```python
from build123d import *

# Parameters (mm, degrees)
F1_DEPTH = 6.858
F2_R     = 2.54
F3_R     = 1.723698
F4_DEPTH = 13.6906


with BuildPart() as f1:
    # F0 (on Top) → F1 (new body)
    with BuildSketch(Plane.XY):
        Polygon((-21.122105, 0), (0, 0), (21.122105, 0), (21.122105, 49.931053), (13.769474, 49.931053), (13.769474, 6.35), (0, 6.35), (-13.769474, 6.35), (-13.769474, 49.931053), (-21.122105, 49.931053), align=None)
    extrude(amount=F1_DEPTH)

    # F2
    f2_edges = [f1.edges().sort_by_distance(p)[0] for p in [
        (13.769474, 28.140527, 0),
        (0, 6.35, 0),
        (-13.769474, 28.140527, 0),
        (0, 0, 6.858),
        (21.122105, 0, 3.429),
        (21.122105, 49.931053, 3.429),
        (21.122105, 24.965527, 6.858),
        (-21.122105, 0, 3.429),
        (-21.122105, 24.965527, 0),
        (-21.122105, 24.965527, 6.858),
        (0, 0, 0),
        (21.122105, 24.965527, 0),
        (-13.769474, 28.140527, 6.858),
        (0, 6.35, 6.858),
    ]]
    fillet(f2_edges, radius=F2_R)

    # F3 (on face) → F4 (join)
    with BuildSketch(Plane(origin=(0, 49.931053, 0), x_dir=(-1, 0, 0), z_dir=(0, 1, 0))):
        with Locations((17.637752, 3.690227)):
            Circle(F3_R)
    extrude(amount=-F4_DEPTH)


solid = f1.part
```
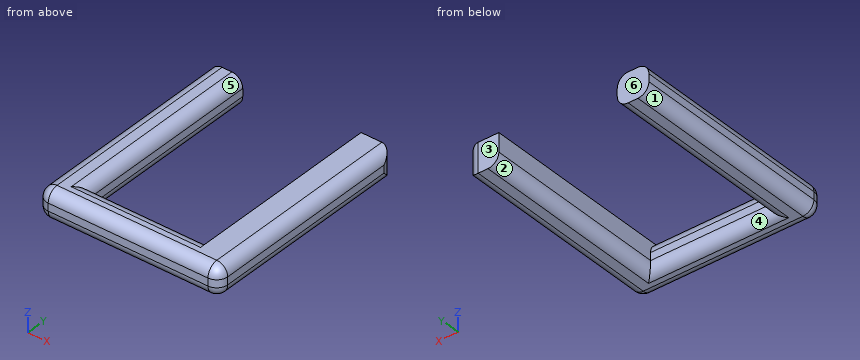
Design review of the part built by this model. Coordinates are the model's own, in mm. Face numbers are marked on the shaded views. A direction names the side the tool comes from. Round coordinates to 2 decimals unless told otherwise and drop trailing zeros. Write each loop counter-clockwise with the first axis right and the second up, starting at its lowest first coordinate (ties: lowest second). Pieces come first, ordered by that corner, then holes.
Item 1: We need section D-D on z = 5. Write out the cut boundary in (x, y), and give its area (3 significant figures).
Item 2: Clearance check with flat-ended pins moving along their axes: pin 1 Ø8 at (x, y) = (12, 36.5) entering from -Z; pin 2 Ø0.5 at (x, z) = (6.5, 4) entering from +Y. State where each tip first meets the part, or that it passes through.
Item 3: The part is to be moulded in two halves that separate along X. For the marked faces 1, 2 and 3, say which applies: +X half, -X half, draft (parallel to the pull), parting line (faces both ways), or undercut.
Item 4: We need section A-A on y = 12. Write out the cut boundary in (x, z).
Item 5: We need section C-C on x = 3.5. Write out the cut boundary in (y, z).
Item 6: For probe 1 along X at (y, z) = (33, 4.25); probe 2 along Y at (x, z) = (2.5, 3.25); probe 3 along X at (y, z) = (8.5, 0.5), list the stretches that pass through material, from the lowest coordinate up.
Item 7: For the marked faces 4, 5 and 6, list the 3-axis set-ups (+Z, -Z, +X, -X, +Y, -Y) from which the entire face can be reached by the end or side of a thin tool; tool diameter is ignored.
Item 8: We need section B-B on z = 2. Write out the cut boundary in (x, y), and give its area (3 significant figures).
Returned:
1. outline: (-21.03, 2.54) arc R2.45 ccw to (-18.58, 0.09) - (18.58, 0.09) arc R2.45 ccw to (21.03, 2.54) - (21.03, 48.07) arc R2.54 ccw to (18.58, 49.93) - (13.77, 49.93) - (13.77, 6.26) - (-13.86, 6.26) - (-13.86, 49.93) - (-21.03, 49.93) - close
1. area: 885 mm2
2. pin 1: stops at z = 0.02
2. pin 2: stops at y = 6.35
3. face 1: -X half
3. face 2: undercut
3. face 3: draft
4. outline: (-21.12, 2.54) arc R2.54 ccw to (-18.58, 0) - (-16.31, 0) arc R2.54 ccw to (-13.77, 2.54) - (-13.77, 4.32) arc R2.54 ccw to (-16.31, 6.86) - (-18.58, 6.86) arc R2.54 ccw to (-21.12, 4.32) - close; (13.77, 2.54) arc R2.54 ccw to (16.31, 0) - (18.58, 0) arc R2.54 ccw to (21.12, 2.54) - (21.12, 4.32) arc R2.54 ccw to (18.58, 6.86) - (13.77, 6.86) - close
5. outline: (0, 2.54) arc R2.54 ccw to (2.54, 0) - (3.81, 0) arc R2.54 ccw to (6.35, 2.54) - (6.35, 4.32) arc R2.54 ccw to (3.81, 6.86) - (2.54, 6.86) arc R2.54 ccw to (0, 4.32) - close
6. probe 1: x = -21.12 to -13.77, 13.77 to 21.12
6. probe 2: y = 0 to 6.35
6. probe 3: x = -20.1 to -14.8, 14.8 to 20.1
7. face 4: -Z, +Y
7. face 5: +Z, +Y
7. face 6: +Z, -Z, +X, -X, +Y
8. outline: (-21.06, 2.54) arc R2.48 ccw to (-18.58, 0.06) - (18.58, 0.06) arc R2.48 ccw to (21.06, 2.54) - (21.06, 47.93) arc R2.54 ccw to (18.58, 49.93) - (13.83, 49.93) - (13.83, 6.29) - (-13.83, 6.29) - (-13.83, 49.93) - (-21.06, 49.93) - close
8. area: 890 mm2
